The model under review builds one solid part; all positions refer to its coordinate system, in mm. Coordinates: 2 decimals unless noted, no trailing zeros. Write each loop counter-clockwise with the first axis right and the second up, starting at its lowest first coordinate (ties: lowest second). Pieces come first, ordered by that corner, then holes.
```python
from build123d import *

# Parameters (mm, degrees)
SKETCH1_R           = 1.5
BOSS_EXTRUDE1_DEPTH = 12
SKETCH2_R           = 2.5
BOSS_EXTRUDE2_DEPTH = 1
DOME1_FACE_RADIUS   = 2.5
DOME1_HEIGHT        = 0.5
SKETCH3_W           = 1.125
SKETCH3_H           = 0.75
SKETCH3_W_2         = 0.75
SKETCH3_H_2         = 1.125
CUT_EXTRUDE1_DEPTH  = 0.75


with BuildPart() as part:
    # Sketch1 → Boss-Extrude1 (new body)
    with BuildSketch(Plane(origin=(0, 0, 0), x_dir=(1, 0, 0), z_dir=(0, 1, 0))):
        Circle(SKETCH1_R)
    extrude(amount=BOSS_EXTRUDE1_DEPTH)

    # Sketch2 → Boss-Extrude2 (add)
    with BuildSketch(Plane(origin=(0, 12, 0), x_dir=(1, 0, 0), z_dir=(0, 1, 0))):
        Circle(SKETCH2_R)
    extrude(amount=BOSS_EXTRUDE2_DEPTH)

    # Dome1: a dome of height H over a round flat face of radius A is a cap of a sphere of radius (A * A + H * H) / (2 * H)
    dome1_r = (DOME1_FACE_RADIUS * DOME1_FACE_RADIUS + DOME1_HEIGHT * DOME1_HEIGHT) / (2 * DOME1_HEIGHT)
    dome1_base = Plane((0, 13, 0), z_dir=(0, 1, 0))
    with Locations(dome1_base.offset(DOME1_HEIGHT - dome1_r)):
        dome1_ball = Sphere(dome1_r, mode=Mode.PRIVATE)
    add(split(dome1_ball, bisect_by=dome1_base, keep=Keep.TOP, mode=Mode.PRIVATE))

    # Sketch3 → Cut-Extrude1 (cut)
    with BuildSketch(Plane(origin=(0, 13.5, 0), x_dir=(1, 0, 0), z_dir=(0, 1, 0))):
        with Locations((-0.9375, 0)):
            Rectangle(SKETCH3_W, SKETCH3_H)
        Rectangle(SKETCH3_W_2, SKETCH3_H)
        with Locations((0, 0.9375)):
            Rectangle(SKETCH3_W_2, SKETCH3_H_2)
        with Locations((0.9375, 0)):
            Rectangle(SKETCH3_W, SKETCH3_H)
        with Locations((0, -0.9375)):
            Rectangle(SKETCH3_W_2, SKETCH3_H_2)
    extrude(amount=-CUT_EXTRUDE1_DEPTH, mode=Mode.SUBTRACT)


solid = part.part
```
Item 1: Take a section at D-D, the plane z = 2. Write out the cut boundary in (x, y).
Solved:
outline: (-1.5, 12) - (1.5, 12) - (1.5, 13) arc R6.18 ccw to (-1.5, 13) - close
Item 2: Take a section at B-B, the plane z = 0. Write out the cut boundary in (x, y).
Solved:
outline: (-2.5, 12) - (-1.5, 12) - (-1.5, 0) - (1.5, 0) - (1.5, 12) - (2.5, 12) - (2.5, 13) arc R6.5 ccw to (1.5, 13.32) - (1.5, 12.75) - (-1.5, 12.75) - (-1.5, 13.32) arc R6.5 ccw to (-2.5, 13) - close
Item 3: Take a section at C-C, the plane y = 6. Write out the cut boundary in (x, z).
Solved:
outline: circle Ø3 at (0, 0)
Item 4: For pin 1 (0.6 mm diameter, centred on y = 13, z = 1, fed in from -X); pin 2 (0.6 mm diameter, centred on y = 13, z = 1, fed in from +X); pin 3 (2 mm diameter, centred on y = 3, z = 2, fed in from +X), all flat-tipped, find the tip position at first contact; note any pin that passes through.
Solved:
pin 1: stops at x = -2.4
pin 2: stops at x = 2.4
pin 3: stops at x = 1.12
Item 5: Take a section at A-A, the plane x = 0. Write out the cut boundary in (y, z).
Solved:
outline: (0, -1.5) - (12, -1.5) - (12, -2.5) - (13, -2.5) arc R6.5 ccw to (13.32, -1.5) - (12.75, -1.5) - (12.75, 1.5) - (13.32, 1.5) arc R6.5 ccw to (13, 2.5) - (12, 2.5) - (12, 1.5) - (0, 1.5) - close
Item 6: To check wall thickness, follow line 1 along Y through (x, z) = (2.2, 1.1); line 2 along Y through (x, z) = (2.25, -0.55); line 3 along X through (y, z) = (3.75, -0.9). State the ranges of each line that lie inside material, in increasing order.
Solved:
line 1: y = 12 to 13.02
line 2: y = 12 to 13.07
line 3: x = -1.2 to 1.2
Item 7: Mouldability with a two-part tool opening along Z and no side actions: class faces 1 (the face through (0, 0, 0)), 2 (the face through (0, 12.75, 0)), 3 (the face through (-0.54, 12.49, 2.44)) as pulls with the +Z half, pulls with the -Z half, needs draft (parallel to the pull), parting line crosses it, or undercut.
Solved:
face 1: needs draft
face 2: undercut
face 3: parting line crosses it
